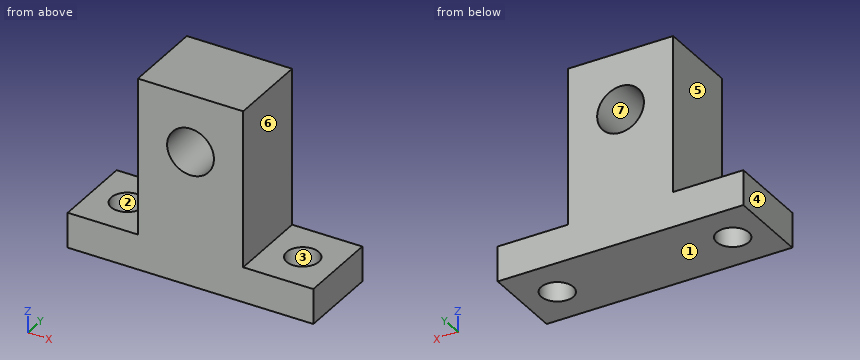
```python
from build123d import *

# Parameters (mm, degrees)
PROFILE_EXTRUDE_DEPTH   = 14
BORE_SKETCH_R           = 4
BORE_CUT_DEPTH          = 15
MOUNTING_HOLE_SKETCH_R  = 2.75
MOUNTING_HOLE_CUT_DEPTH = 7


with BuildPart() as part:
    # Profile Sketch → Profile Extrude (new body)
    with BuildSketch(Plane(origin=(0, 0, 0), x_dir=(1, 0, 0), z_dir=(0, 1, 0))):
        Polygon((9, -3), (21, -3), (21, 3), (-21, 3), (-21, -3), (-9, -3), (-9, -29.8), (9, -29.8), align=None)
    extrude(amount=PROFILE_EXTRUDE_DEPTH)

    # Bore Sketch → Bore Cut (cut, through all)
    with BuildSketch(Plane.XZ):
        with Locations((0, 20)):
            Circle(BORE_SKETCH_R)
    extrude(amount=-BORE_CUT_DEPTH, mode=Mode.SUBTRACT)

    # Mounting Hole Sketch → Mounting Hole Cut (cut, through all)
    with BuildSketch(Plane.XY.offset(3)):
        with Locations((15, 7)):
            Circle(MOUNTING_HOLE_SKETCH_R)
        with Locations((-15, 7)):
            Circle(MOUNTING_HOLE_SKETCH_R)
    extrude(amount=-MOUNTING_HOLE_CUT_DEPTH, mode=Mode.SUBTRACT)


solid = part.part
```
Input: part model. Units: mm. Frame: model coordinates. Face numbers are marked on the shaded views. A direction names the side the tool comes from. Round coordinates to 2 decimals unless told otherwise and drop trailing zeros. Loops run counter-clockwise (first coordinate to the right, second up) from the corner with the lowest first, then second, coordinate; pieces in that order, holes last. Notation, with made-up numbers: (89, 1) -> (133, 1) arc R18 cw to (133, 33) -> close; hole circle Ø11 at (72, 73.25). An arc over 180 degrees is marked (long way). Use one line per item in the form item = value. Start each with the question number.
Item 1: Section query C-C on z = 20. Return the cut outline in (x, y), then the cut area to 3 significant figures.
Item 2: Set-up query: the marked faces 5, 6 and 7. Return all of +Z, -Z, +X, -X, +Y, -Y with unobstructed straight access to the full face (end or side cutting, diameter ignored); none if empty.
Item 3: Mould query, pull axis X, two halves, no side actions, for the marked faces 1, 2, 3 and 4. Classes: pulls with the +X half, pulls with the -X half, needs draft (parallel to the pull), parting line crosses it, or undercut.
Item 4: Section query B-B on x = -15. Return the cut outline in (y, z).
Item 5: Section query A-A on y = 7. Return the cut outline in (x, z), then the cut area to 3 significant figures.
Item 6: Material intervals for L1, parallel to Y at x = 15, z = 0; L2, parallel to Z at x = 0, y = 4.75; L3, parallel to Z at x = -10, y = 13, sorted ascending. Write a range as from..to.
Item 7: Contact query for flat-ended pins moving along their axis: pin 1 Ø5 at (x, z) = (0, 20) entering from -Y; pin 2 Ø1.5 at (y, z) = (4, 6.5) entering from -X; pin 3 Ø6 at (x, y) = (13.5, 7.5) entering from +Z; pin 4 Ø1.5 at (y, z) = (11, 23) entering from +X. Output: stop coordinate, or through.
Item 8: Section query D-D on y = 11.75. Return the cut outline in (x, z).
Ans:
q1.outline = (-9, 0) -> (-4, 0) -> (-4, 14) -> (-9, 14) -> close; (4, 0) -> (9, 0) -> (9, 14) -> (4, 14) -> close
q1.area = 140 mm^2
q2.face_5 = +Z, -X, +Y, -Y
q2.face_6 = +Z, +X, +Y, -Y
q2.face_7 = +Y, -Y
q3.face_1 = needs draft
q3.face_2 = undercut
q3.face_3 = undercut
q3.face_4 = pulls with the -X half
q4.outline = (0, -3) -> (4.25, -3) -> (4.25, 3) -> (0, 3) -> close; (9.75, -3) -> (14, -3) -> (14, 3) -> (9.75, 3) -> close
q5.outline = (-21, -3) -> (-17.75, -3) -> (-17.75, 3) -> (-21, 3) -> close; (-12.25, -3) -> (12.25, -3) -> (12.25, 3) -> (9, 3) -> (9, 29.8) -> (-9, 29.8) -> (-9, 3) -> (-12.25, 3) -> close; (17.75, -3) -> (21, -3) -> (21, 3) -> (17.75, 3) -> close; hole circle Ø8 at (0, 20)
q5.area = 618 mm^2
q6.L1 = 0..4.25, 9.75..14
q6.L2 = -3..16, 24..29.8
q6.L3 = -3..3
q7.pin_1 = through
q7.pin_2 = -9
q7.pin_3 = 3
q7.pin_4 = 9
q8.outline = (-21, -3) -> (21, -3) -> (21, 3) -> (9, 3) -> (9, 29.8) -> (-9, 29.8) -> (-9, 3) -> (-21, 3) -> close; hole circle Ø8 at (0, 20)
